from build123d import *

# Parameters (mm, degrees)
F0_W     = 120
F0_H     = 46
F1_DEPTH = 2
F2_W     = 120
F2_H     = 46
F3_DEPTH = 5
F4_R     = 3
F5_R     = 1
F6_DEPTH = 25


with BuildPart() as f1:
    # F0 (on Top) → F1 (new body)
    with BuildSketch(Plane.XY):
        Rectangle(F0_W, F0_H)
    extrude(amount=F1_DEPTH)

    # F2 (on face) → F3 (join)
    with BuildSketch(Plane.XY.offset(2)):
        Rectangle(F2_W, F2_H)
        Polygon((58, 21), (58, -21), (-57.0000000355, -21), (-58, -21), (-58, -20), (-58, -18), (-58, 21), align=None, mode=Mode.SUBTRACT)
    extrude(amount=F3_DEPTH)

    # F4
    f4_edges = [f1.edges().sort_by_distance(p)[0] for p in [
        (-60, 23, 3.5),
        (-60, -23, 3.5),
        (60, 23, 3.5),
        (60, -23, 3.5),
    ]]
    fillet(f4_edges, radius=F4_R)

    # F5
    f5_edges = [f1.edges().sort_by_distance(p)[0] for p in [
        (0, 23, 0),
        (-59.12132, 22.12132, 0),
        (-60, 0, 0),
        (-59.12132, -22.12132, 0),
        (0, -23, 0),
        (60, 0, 0),
        (59.12132, 22.12132, 0),
        (59.12132, -22.12132, 0),
    ]]
    fillet(f5_edges, radius=F5_R)

    # F2 (on face) → F6 (cut)
    with BuildSketch(Plane.XY.offset(2)):
        with BuildLine():
            ThreePointArc((-56, -18), (-57, -17), (-58, -18))
            ThreePointArc((-58, -18), (-57.7071067812, -18.7071067812), (-57, -19))
            ThreePointArc((-57, -19), (-56.2928932188, -18.7071067812), (-56, -18))
        make_face()
        with BuildLine():
            ThreePointArc((-57, -19), (-56.2928932188, -19.2928932188), (-56, -20))
            Line((-56, -20), (-56, -18))
            ThreePointArc((-56, -18), (-56.2928932188, -18.7071067812), (-57, -19))
        make_face()
        with BuildLine():
            Line((-58, -18), (-58, -20))
            ThreePointArc((-58, -20), (-57.7071067812, -19.2928932188), (-57, -19))
            ThreePointArc((-57, -19), (-57.7071067812, -18.7071067812), (-58, -18))
        make_face()
        with BuildLine():
            ThreePointArc((-58, -20), (-57.7071067937, -20.7071067687), (-57.0000000355, -21))
            ThreePointArc((-57.0000000355, -21), (-56.2928932313, -20.7071067937), (-56, -20))
            ThreePointArc((-56, -20), (-56.2928932188, -19.2928932188), (-57, -19))
            ThreePointArc((-57, -19), (-57.7071067812, -19.2928932188), (-58, -20))
        make_face()
    extrude(amount=-F6_DEPTH, mode=Mode.SUBTRACT)


solid = f1.part
Design review of the part built by this model. Coordinates are the model's own, in mm. A direction names the side the tool comes from. Coordinates: 2 decimals unless noted, no trailing zeros. Order: outer loops, then holes, each group sorted by start corner. A loop starts at its lowest first (then second) coordinate and runs counter-clockwise, first axis right, second up.
Item 1: For pin 1 Ø5 at (x, y) = (-39.5, 16.5) entering from +Z; pin 2 Ø2 at (y, z) = (-19.5, 0.5) entering from -X, all flat-tipped, find the tip position at first contact; note any pin that passes through.
Item 2: Take a section at A-A, the plane z = 5.5. Write out the cut boundary in (x, y).
Item 3: For line 1 (Y direction, x = -46, z = 5); line 2 (X direction, y = 12, z = 6); line 3 (Z direction, x = -45.5, y = -8), list the stretches that pass through material, from the lowest coordinate up.
Item 4: Take a section at B-B, the plane x = 13.5. Write out the cut boundary in (y, z).
Item 5: The part is to be moulded in two halves that separate along Y. For faces 4 (the flat face through (-56, -19, 1)), 5 (the cylindrical face through (59.14, 22.1, 3.96)), 6 (the flat face through (-60, 0, 4)), say which applies: pulls with the +Y half, pulls with the -Y half, needs draft (parallel to the pull), parting line crosses it, or undercut.
Item 6: For faces 1 (the cylindrical face through (-59.14, 22.1, 3.96)), 2 (the flat face through (-1, 0, 2)), 3 (the cylindrical face through (-57, -17, 1)), list the 3-axis set-ups (+Z, -Z, +X, -X, +Y, -Y) from which the entire face can be reached by the end or side of a thin tool; tool diameter is ignored.
Item 7: Take a section at C-C, the plane y = -3.5. Write out the cut boundary in (x, z), then the cut area to 3 significant figures.
The answers:
1. pin 1: stops at z = 2
1. pin 2: stops at x = -60
2. outline: (-60, -20) arc R3 ccw to (-57, -23) - (57, -23) arc R3 ccw to (60, -20) - (60, 20) arc R3 ccw to (57, 23) - (-57, 23) arc R3 ccw to (-60, 20) - close; hole (-58, -21) - (58, -21) - (58, 21) - (-58, 21) - close
3. line 1: y = -23 to -21, 21 to 23
3. line 2: x = -60 to -58, 58 to 60
3. line 3: z = 0 to 2
4. outline: (-23, 1) arc R1 ccw to (-22, 0) - (22, 0) arc R1 ccw to (23, 1) - (23, 7) - (21, 7) - (21, 2) - (-21, 2) - (-21, 7) - (-23, 7) - close
5. face 4: undercut
5. face 5: pulls with the +Y half
5. face 6: needs draft
6. face 1: +Z, -Z, -X, +Y
6. face 2: +Z
6. face 3: +Z, -Z
7. outline: (-60, 1) arc R1 ccw to (-59, 0) - (59, 0) arc R1 ccw to (60, 1) - (60, 7) - (58, 7) - (58, 2) - (-58, 2) - (-58, 7) - (-60, 7) - close
7. area: 260 mm2
